Geometry: final body of the model. Coordinates: model frame, mm. Face numbers are marked on the shaded views. A direction names the side the tool comes from. Give positions to 0.01 mm unless a question says otherwise; leave off trailing zeros. Write each loop counter-clockwise with the first axis right and the second up, starting at its lowest first coordinate (ties: lowest second). Pieces come first, ordered by that corner, then holes.
Q1. Line query: line 1 (X direction, y = 3.5, z = 16); line 2 (X direction, y = 7.25, z = -17.5); line 3 (Z direction, x = -5, y = 5.25). Output: solid intervals per line, ascending.
Q2. Section A-A (y = 4). Return the cut outline in (x, z), plus the area to 3 significant figures.
Q3. Section D-D (z = 15.5). Return the cut outline in (x, y), plus the area to 3 significant figures.
Q4. Section B-B (z = -5). Return the cut outline in (x, y).
Q5. Reachability of the marked faces 4, 5 and 6 from +Z, -Z, +X, -X, +Y, -Y: full face, straight path, thin tool, end or side. Return the list, or none.
Q6. Mould query, pull axis Z, two halves, no side actions, for the marked faces 1, 2 and 3. Classes: +Z half, -Z half, draft (parallel to the pull), parting line (faces both ways), or undercut.
Q7. Section C-C (y = 6.75). Return the cut outline in (x, z).
Q8. Pin query (flat end, axial travel): pin 1 Ø2 at (y, z) = (4, -4) entering from +X; pin 2 Ø4 at (y, z) = (3, -5) entering from -X; pin 3 Ø3 at (y, z) = (4, 5) entering from +X; pin 4 Ø2 at (y, z) = (5.5, 11.5) entering from +X. Return the tip coordinate at first contact, or that it passes through.
from build123d import *

# Parameters (mm, degrees)
SKETCH1_R           = 1.7
SKETCH1_W           = 6
SKETCH1_H           = 20
BOSS_EXTRUDE1_DEPTH = 7.5
SKETCH3_R           = 1.7
CUT_EXTRUDE2_DEPTH  = 6
FILLET1_R           = 2


with BuildPart() as part:
    # Sketch1 → Boss-Extrude1 (new body)
    # profile 1 of 3: a face of its own
    with BuildSketch(Plane(origin=(0, 0, 0), x_dir=(1, 0, 0), z_dir=(0, 1, 0))):
        Polygon((-3, -10), (3, -10), (9, -14), (9, -20), (-9, -20), (-9, -14), align=None)
        with Locations(Location((4, -16, 0), (0, 0, 270))):
            Circle(SKETCH1_R, mode=Mode.SUBTRACT)
        with Locations(Location((-4, -16, 0), (0, 0, 270))):
            Circle(SKETCH1_R, mode=Mode.SUBTRACT)
    # profile 2 of 3: a face of its own
    with BuildSketch(Plane(origin=(0, 0, 0), x_dir=(1, 0, 0), z_dir=(0, 1, 0))):
        Rectangle(SKETCH1_W, SKETCH1_H)
    # profile 3 of 3: a face of its own
    with BuildSketch(Plane(origin=(0, 0, 0), x_dir=(1, 0, 0), z_dir=(0, 1, 0))):
        Polygon((9, 14), (3, 10), (-3, 10), (-9, 14), (-9, 20), (9, 20), align=None)
        with Locations(Location((4, 16, 0), (0, 0, 270))):
            Circle(SKETCH1_R, mode=Mode.SUBTRACT)
        with Locations(Location((-4, 16, 0), (0, 0, 270))):
            Circle(SKETCH1_R, mode=Mode.SUBTRACT)
    extrude(amount=BOSS_EXTRUDE1_DEPTH)

    # Sketch3 → Cut-Extrude2 (cut)
    with BuildSketch(Plane(origin=(3, 0, 0), x_dir=(0, 0, -1), z_dir=(1, 0, 0))):
        with Locations((-5, 4)):
            Circle(SKETCH3_R)
        with Locations((5, 4)):
            Circle(SKETCH3_R)
    extrude(amount=-CUT_EXTRUDE2_DEPTH, mode=Mode.SUBTRACT)

    # Fillet1
    fillet1_edges = [part.edges().sort_by_distance(p)[0] for p in [
        (-9, 3.75, -20),
    ]]
    fillet(fillet1_edges, radius=FILLET1_R)


solid = part.part
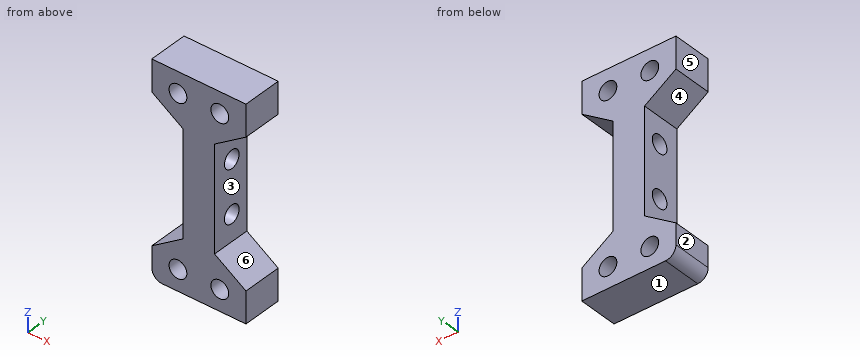
Computed:
1. line 1: x = -9 to -5.7, -2.3 to 2.3, 5.7 to 9
1. line 2: x = -9 to -4.8, -3.2 to 3.2, 4.8 to 9
1. line 3: z = -20 to -17.37, -14.63 to -11.33, 11.33 to 14.63, 17.37 to 20
2. outline: (-9, -18) arc R2 ccw to (-7, -20) - (9, -20) - (9, -14) - (3, -10) - (3, -6.7) - (-3, -6.7) - (-3, -10) - (-9, -14) - close; (-9, 14) - (-3, 10) - (-3, 6.7) - (3, 6.7) - (3, 10) - (9, 14) - (9, 20) - (-9, 20) - close; (-3, -3.3) - (3, -3.3) - (3, 3.3) - (-3, 3.3) - close; hole circle Ø3.4 at (-4, -16); hole circle Ø3.4 at (-4, 16); hole circle Ø3.4 at (4, -16); hole circle Ø3.4 at (4, 16)
2. area: 354 mm2
3. outline: (-9, 0) - (-5.62, 0) - (-5.62, 7.5) - (-9, 7.5) - close; (-2.38, 0) - (2.38, 0) - (2.38, 7.5) - (-2.38, 7.5) - close; (5.62, 0) - (9, 0) - (9, 7.5) - (5.62, 7.5) - close
3. area: 86.3 mm2
4. outline: (-3, 0) - (3, 0) - (3, 2.3) - (-3, 2.3) - close; (-3, 5.7) - (3, 5.7) - (3, 7.5) - (-3, 7.5) - close
5. face 4: -X, +Y, -Y
5. face 5: +Z, -Z, -X, +Y, -Y
5. face 6: +X, +Y, -Y
6. face 1: -Z half
6. face 2: draft
6. face 3: undercut
7. outline: (-9, -18) arc R2 ccw to (-7, -20) - (9, -20) - (9, -14) - (3, -10) - (3, 10) - (9, 14) - (9, 20) - (-9, 20) - (-9, 14) - (-3, 10) - (-3, -10) - (-9, -14) - close; hole circle Ø3.4 at (-4, -16); hole circle Ø3.4 at (-4, 16); hole circle Ø3.4 at (4, -16); hole circle Ø3.4 at (4, 16)
8. pin 1: stops at x = 3
8. pin 2: stops at x = -3
8. pin 3: passes through
8. pin 4: stops at x = 6.75
